Read the model definition and answer for the solid it produces. Units are mm, in the model's axes. Face numbers are marked on the shaded views. A direction names the side the tool comes from. Give positions to 0.01 mm unless a question says otherwise; leave off trailing zeros. Order: outer loops, then holes, each group sorted by start corner. A loop starts at its lowest first (then second) coordinate and runs counter-clockwise, first axis right, second up.
Item 1: A cutting plane is placed at B-B (z = -5.25). Write down the section's boundary in (x, y).
Item 2: Find the intervals of material crossed by line 1 along Z through (x, y) = (-0.8, 1); line 2 along Z through (x, y) = (1.5, 0.5); line 3 along X through (y, z) = (-0.25, 2.5), in increasing order.
Item 3: Which of the six approach directions +Z, -Z, +X, -X, +Y, -Y give full straight-line access (tool end or side, diameter ignored) to the marked faces 4 and 5?
Item 4: A cutting plane is placed at A-A (z = 1.5). Write down the section's boundary in (x, y).
Item 5: The mould has two halves that part along X. Classify the marked faces 1, 2 and 3: +X half, -X half, draft (parallel to the pull), parting line (faces both ways), or undercut.
Item 6: A cutting plane is placed at C-C (y = 0). Write down the section's boundary in (x, z), plus the area to 3 significant figures.
Item 7: Given pin 1 Ø2 at (x, z) = (-2, 1.5) entering from +Y; pin 2 Ø2 at (x, z) = (0.5, 4.5) entering from -Y; pin 3 Ø2.5 at (x, y) = (0, 0) entering from +Z, each flat-ended and moving along its own axis, determine where each tip first touches the part or whether it passes through.
from build123d import *

# Parameters (mm, degrees)
PAD_DEPTH    = 10
SKETCH001_R  = 1.5
POCKET_DEPTH = 15
SKETCH002_R  = 1.5
PAD001_DEPTH = 5.5


with BuildPart() as part:
    # Sketch → Pad (new body, symmetric)
    with BuildSketch(Plane.XY):
        Polygon((2.6, 1.501111), (0, 3.002221), (-2.6, 1.501111), (-2.6, -1.501111), (0, -3.002221), (2.6, -1.501111), align=None)
    extrude(amount=PAD_DEPTH, both=True)

    # Sketch001 (on Face8 of Pad) → Pocket (cut)
    with BuildSketch(Plane.XY.offset(10)):
        Circle(SKETCH001_R)
    extrude(amount=-POCKET_DEPTH, mode=Mode.SUBTRACT)

    # Sketch002 (on Face4 of Pocket) → Pad001 (join)
    with BuildSketch(Plane(origin=(0, 0, -10), x_dir=(1, 0, 0), z_dir=(0, 0, -1))):
        Circle(SKETCH002_R)
    extrude(amount=PAD001_DEPTH)

    # Sketch004 → Groove (revolve, cut)
    with BuildSketch(Plane.YZ):
        Polygon((2, 10.5), (5, 10.5), (5, -10.5), (2, -10.5), (3.27, -9.23), (3.27, 9.23), align=None)
    revolve(axis=Axis((0, 0, 0), (0, 0, 1)), mode=Mode.SUBTRACT)


solid = part.part
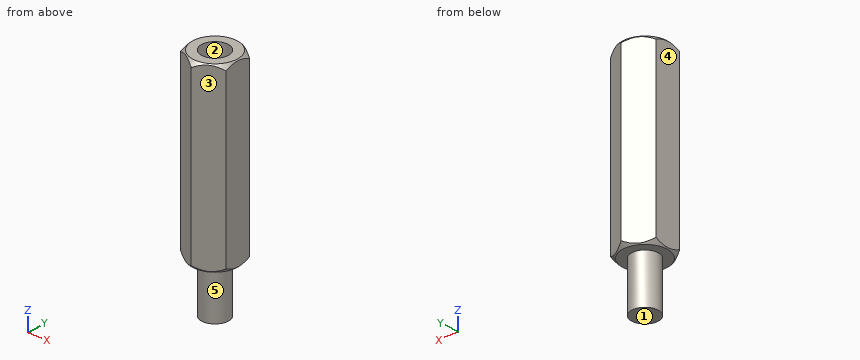
Response values:
1. outline: (-2.6, -1.5) - (0, -3) - (2.6, -1.5) - (2.6, 1.5) - (0, 3) - (-2.6, 1.5) - close
2. line 1: z = -15.5 to -5
2. line 2: z = -10 to 10
2. line 3: x = -2.6 to -1.48, 1.48 to 2.6
3. face 4: +Z, -Z, -X, +Y, -Y
3. face 5: -Z
4. outline: (-2.6, -1.5) - (0, -3) - (2.6, -1.5) - (2.6, 1.5) - (0, 3) - (-2.6, 1.5) - close; hole circle Ø3 at (0, 0)
5. face 1: draft
5. face 2: undercut
5. face 3: +X half
6. outline: (-2.6, -9.9) - (-2.5, -10) - (-1.5, -10) - (-1.5, -15.5) - (1.5, -15.5) - (1.5, -10) - (2.5, -10) - (2.6, -9.9) - (2.6, 9.9) - (2.5, 10) - (1.5, 10) - (1.5, -5) - (-1.5, -5) - (-1.5, 10) - (-2.5, 10) - (-2.6, 9.9) - close
6. area: 75.5 mm2
7. pin 1: stops at y = 2.42
7. pin 2: stops at y = -3
7. pin 3: stops at z = -5
